Read the model definition and answer for the solid it produces. Units are mm, in the model's axes. Face numbers are marked on the shaded views. A direction names the side the tool comes from. Give positions to 0.01 mm unless a question says otherwise; leave off trailing zeros. Order: outer loops, then holes, each group sorted by start corner. A loop starts at its lowest first (then second) coordinate and runs counter-clockwise, first axis right, second up.
```python
from build123d import *

# Parameters (mm, degrees)
ESQUISSE1_R             = 3.15
ESQUISSE1_R_2           = 2
BOSS_EXTRU_1_DEPTH      = 1.6
ESQUISSE2_R             = 9.5
ESQUISSE2_R_2           = 3.15
BOSS_EXTRU_2_DEPTH      = 9.5
CONG_1_R                = 1
BOSS_EXTRU_3_DEPTH      = 13
ESQUISSE4_R             = 2
ENL_V_MAT_EXTRU_1_DEPTH = 19.5


with BuildPart() as part:
    # Esquisse1 → Boss.-Extru.1 (new body)
    with BuildSketch(Plane(origin=(0, 0, 0), x_dir=(1, 0, 0), z_dir=(0, 1, 0))):
        with BuildLine():
            Line((0, 11.5), (-25, 11.5))
            ThreePointArc((-25, 11.5), (-31.5, 5), (-25, -1.5))
            Line((-25, -1.5), (-16.90921754, -1.5))
            ThreePointArc((-16.90921754, -1.5), (-13.826301978, -3.956560509), (-15.532463951, -7.510159982))
            Line((-15.532463951, -7.510159982), (-17.532463951, -8.477187494))
            Line((-17.532463951, -8.477187494), (-13, -18.5))
            Line((-13, -18.5), (4.73848504, -10.478394893))
            ThreePointArc((4.73848504, -10.478394893), (11.241697854, 2.423680954), (0, 11.5))
        make_face()
        Circle(ESQUISSE1_R, mode=Mode.SUBTRACT)
        with Locations((-25, 5)):
            Circle(ESQUISSE1_R_2, mode=Mode.SUBTRACT)
    extrude(amount=BOSS_EXTRU_1_DEPTH)

    # Esquisse2 → Boss.-Extru.2 (add)
    with BuildSketch(Plane(origin=(0, 1.6, 0), x_dir=(1, 0, 0), z_dir=(0, 1, 0))):
        Circle(ESQUISSE2_R)
        Circle(ESQUISSE2_R_2, mode=Mode.SUBTRACT)
    extrude(amount=BOSS_EXTRU_2_DEPTH)

    # Congé1
    cong_1_edges = [part.edges().sort_by_distance(p)[0] for p in [
        (-9.5, 11.1, 0),
    ]]
    fillet(cong_1_edges, radius=CONG_1_R)

    # Esquisse3 → Boss.-Extru.3 (add)
    with BuildSketch(Plane(origin=(0, 1.6, 0), x_dir=(1, 0, 0), z_dir=(0, 1, 0))):
        Polygon((-17.532463951, -8.477187494), (-13, -18.5), (-11.633703391, -17.88214048), (-16.182035998, -7.824237002), align=None)
    extrude(amount=BOSS_EXTRU_3_DEPTH)

    # Esquisse4 → Enlèv. mat.-Extru.1 (cut, through all)
    with BuildSketch(Plane.XY):
        with Locations((0, 6)):
            Circle(ESQUISSE4_R)
    extrude(amount=ENL_V_MAT_EXTRU_1_DEPTH, mode=Mode.SUBTRACT)


solid = part.part
```
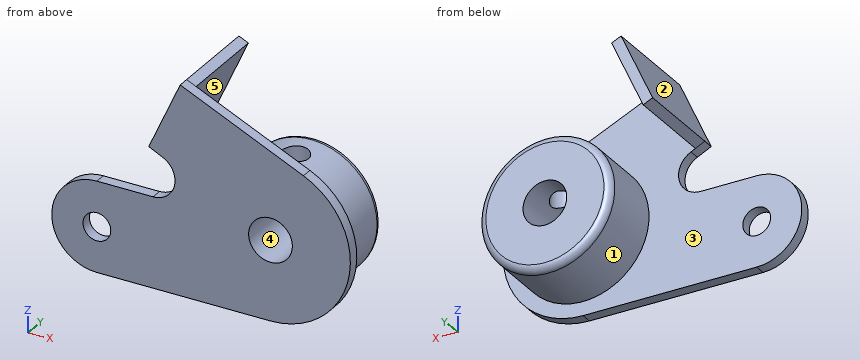
1) The part is cut by section B-B on y = 6. Determine the outline of the cut face in (x, z), and give its area (3 significant figures).
Final values:
outline: (-17.53, 8.48) - (-16.18, 7.82) - (-11.63, 17.88) - (-13, 18.5) - close; (-2, 2.43) - (-2, 9.29) arc R9.5 ccw (long way) to (2, 9.29) - (2, 2.43) arc R3.15 cw (long way) to start
area: 243 mm2
2) Given pin 1 (2.5 mm diameter, centred on x = 0, y = 6, fed in from -Z); pin 2 (10 mm diameter, centred on x = -10, z = 3, fed in from +Y); pin 3 (6 mm diameter, centred on x = -20, y = 5.5, fed in from +Z); pin 4 (2.5 mm diameter, centred on x = -25, z = -5, fed in from -Y), each flat-ended and moving along its own axis, determine where each tip first touches the part or whether it passes through.
Final values:
pin 1: stops at z = -9.5
pin 2: stops at y = 11.1
pin 3: stops at z = 9.65
pin 4: passes through
3) The part is cut by section C-C on x = -27.5. Determine the outline of the cut face in (y, z).
Final values:
outline: (0, -11) - (1.6, -11) - (1.6, 1) - (0, 1) - close
4) Consider L1, parallel to Z at x = -25, y = 1.1; L2, parallel to X at y = 5.5, z = 0; L3, parallel to Y at x = 0, z = 5.25. Determine where each line is inside the solid, lowest interval first.
Final values:
L1: z = -11.5 to -7, -3 to 1.5
L2: x = -9.5 to -3.15, 3.15 to 9.5
L3: y = 0 to 4, 8 to 11.1
5) The part is cut by section D-D on y = 13. Determine the outline of the cut face in (x, z).
Final values:
outline: (-17.53, 8.48) - (-16.18, 7.82) - (-11.63, 17.88) - (-13, 18.5) - close
6) A tool of negligible diameter and unlimited length cuts with its end or side. For the marked faces 1 and 2, from which of +Z, -Z, +X, -X, +Y, -Y can it reach the whole face along a straight path? Write none if from no direction.
Final values:
face 1: +Y
face 2: +Z, -X, +Y, -Y
7) For a pull along Z with two mould halves and no side action, classify the marked faces 3, 4 and 5 as released by +Z, released by -Z, zero draft, split by the parting line, or undercut.
Final values:
face 3: zero draft
face 4: undercut
face 5: released by -Z
8) The part is cut by section A-A on z = 0. Determine the outline of the cut face in (x, y).
Final values:
outline: (-29.15, 0) - (-3.15, 0) - (-3.15, 11.1) - (-8.5, 11.1) arc R1 ccw to (-9.5, 10.1) - (-9.5, 1.6) - (-29.15, 1.6) - close; (3.15, 0) - (11.5, 0) - (11.5, 1.6) - (9.5, 1.6) - (9.5, 10.1) arc R1 ccw to (8.5, 11.1) - (3.15, 11.1) - close
